The model under review builds one solid part; all positions refer to its coordinate system, in mm. Coordinates: 2 decimals unless noted, no trailing zeros. Write each loop counter-clockwise with the first axis right and the second up, starting at its lowest first coordinate (ties: lowest second). Pieces come first, ordered by that corner, then holes.
```python
from build123d import *

# Parameters (mm, degrees)
SKETCH_1_R           = 5
EXTRUDE_1_DEPTH      = 26
EXTRUDE_START        = 85
SKETCH_3_R           = 5
EXTRUDE_3_DEPTH      = 85
EXTRUDE_4_REACH      = 87.889
EXTRUDE_4_END_RADIUS = 5


with BuildPart() as part:
    # 草图1 → 凸台-拉伸1 (new body)
    with BuildSketch(Plane.XY):
        with Locations(Location((0, 0, 0), (0, 0, 180))):
            Circle(SKETCH_1_R)
    extrude(amount=EXTRUDE_1_DEPTH)

    # 草图3 → 凸台-拉伸3 (add)
    with BuildSketch(Plane(origin=(0, 0, 0), x_dir=(-1, 0, 0), z_dir=(0, 0, -1)).offset(EXTRUDE_START)):
        Circle(SKETCH_3_R)
    extrude(amount=-EXTRUDE_3_DEPTH)

    # 凸台-拉伸4: up to this cylinder (the profile starts outside it)
    extrude_4_end = Plane(origin=(0, 0, 13), z_dir=(0, 0, -1)) * Cylinder(EXTRUDE_4_END_RADIUS, 186.778, mode=Mode.PRIVATE)
    # 草图5 → 凸台-拉伸4 (add, up to the surface)
    with BuildSketch(Plane(origin=(0, 6.269, 0), x_dir=(1, 0, 0), z_dir=(0, 1, 0)), mode=Mode.PRIVATE) as extrude_4_sk1:
        with BuildLine():
            Line((1.5, -3.5), (1.5, -22.5))
            ThreePointArc((1.5, -22.5), (0, -24), (-1.5, -22.5))
            Line((-1.5, -22.5), (-1.5, -3.5))
            ThreePointArc((-1.5, -3.5), (0, -2), (1.5, -3.5))
        make_face()
    extrude_4_tool1 = extrude(extrude_4_sk1.sketch, amount=-EXTRUDE_4_REACH, mode=Mode.PRIVATE) - extrude_4_end
    add(extrude_4_tool1.solids().sort_by_distance((0, 6.269, 13))[0])


solid = part.part
```
Item 1: Take a section at B-B, the plane z = 8. Write out the cut boundary in (x, y).
Solved:
outline: (-1.5, 4.77) arc R5 ccw (long way) to (1.5, 4.77) - (1.5, 6.27) - (-1.5, 6.27) - close
Item 2: Take a section at C-C, the plane y = -3. Write out the cut boundary in (x, z), plus the area to 3 significant figures.
Solved:
outline: (-4, -85) - (4, -85) - (4, 26) - (-4, 26) - close
area: 888 mm2
Item 3: Take a section at D-D, the plane z = -47. Write out the cut boundary in (x, y), plus the area to 3 significant figures.
Solved:
outline: circle Ø10 at (0, 0)
area: 78.5 mm2
Item 4: Take a section at A-A, the plane x = 0. Write out the cut boundary in (y, z).
Solved:
outline: (-5, -85) - (5, -85) - (5, 2) - (6.27, 2) - (6.27, 24) - (5, 24) - (5, 26) - (-5, 26) - close
Item 5: To check wall thickness, follow line 1 along X through (y, z) = (5, 20.5); line 2 along Y through (x, z) = (3, -58.5); line 3 along X through (y, z) = (-2.25, -50). State the ranges of each line that lie inside material, in increasing order.
Solved:
line 1: x = -1.5 to 1.5
line 2: y = -4 to 4
line 3: x = -4.47 to 4.47
Item 6: For pin 1 (0.7 mm diameter, centred on y = 5.5, z = 16, fed in from +X); pin 2 (4 mm diameter, centred on x = 0, z = -41, fed in from +Y); pin 3 (1.2 mm diameter, centred on y = 5, z = 8.5, fed in from -X); pin 4 (3 mm diameter, centred on x = -1.5, z = -55, fed in from -Y), all flat-tipped, find the tip position at first contact; note any pin that passes through.
Solved:
pin 1: stops at x = 1.5
pin 2: stops at y = 5
pin 3: stops at x = -2.37
pin 4: stops at y = -5
